For this review, take the finished solid that the model builds, in its own axes (mm). Face numbers are marked on the shaded views. A direction names the side the tool comes from. Give positions to 0.01 mm unless a question says otherwise; leave off trailing zeros. Loops run counter-clockwise (first coordinate to the right, second up) from the corner with the lowest first, then second, coordinate; pieces in that order, holes last. Notation, with made-up numbers: (34.5, 46) - (85.5, 46) arc R33 cw to (85.5, 81) - close; hole circle Ø11 at (64, 81.25). An arc over 180 degrees is marked (long way). Answer as CSV lines item,"result".
from build123d import *

# Parameters (mm, degrees)
EXTRUDE_2_DEPTH = 3
SKETCH_4_R      = 2.5
SKETCH_4_R_2    = 0.95
SKETCH_4_R_3    = 0.973149492
EXTRUDE_5_DEPTH = 6
SKETCH_6_W      = 16
SKETCH_6_H      = 8
EXTRUDE_6_DEPTH = 2.5
EXTRUDE_7_DEPTH = 3.8


with BuildPart() as part:
    # Эскиз1 → Бобышка-Вытянуть2 (new body)
    with BuildSketch(Plane(origin=(0, 0, 0), x_dir=(1, 0, 0), z_dir=(0, 1, 0))):
        with BuildLine():
            Line((-21.078452696, 29.831456886), (2.921547304, 29.831456886))
            ThreePointArc((2.921547304, 29.831456886), (5.042867648, 28.95277723), (5.921547304, 26.831456886))
            Line((5.921547304, 26.831456886), (5.921547304, 2.831456886))
            ThreePointArc((5.921547304, 2.831456886), (5.042867648, 0.710136543), (2.921547304, -0.168543114))
            Line((2.921547304, -0.168543114), (-21.078452696, -0.168543114))
            ThreePointArc((-21.078452696, -0.168543114), (-23.19977304, 0.710136543), (-24.078452696, 2.831456886))
            Line((-24.078452696, 2.831456886), (-24.078452696, 26.831456886))
            ThreePointArc((-24.078452696, 26.831456886), (-23.19977304, 28.95277723), (-21.078452696, 29.831456886))
        make_face()
    extrude(amount=EXTRUDE_2_DEPTH)

    # Эскиз4 → Бобышка-Вытянуть5 (add)
    # profile 1 of 4: a face of its own
    with BuildSketch(Plane.XZ):
        with Locations(Location((1.421547304, -4.831456886, 0), (0, 0, 90))):
            Circle(SKETCH_4_R)
        with Locations(Location((1.421547304, -4.831456886, 0), (0, 0, 270))):
            Circle(SKETCH_4_R_2, mode=Mode.SUBTRACT)
    # profile 2 of 4: a face of its own
    with BuildSketch(Plane.XZ):
        with Locations(Location((-19.578452696, -4.831456886, 0), (0, 0, 90))):
            Circle(SKETCH_4_R)
        with Locations(Location((-19.578452696, -4.831456886, 0), (0, 0, 270))):
            Circle(SKETCH_4_R_3, mode=Mode.SUBTRACT)
    # profile 3 of 4: a face of its own
    with BuildSketch(Plane.XZ):
        with Locations(Location((1.421547304, -17.331456886, 0), (0, 0, 90))):
            Circle(SKETCH_4_R)
        with Locations(Location((1.421547304, -17.331456886, 0), (0, 0, 270))):
            Circle(SKETCH_4_R_2, mode=Mode.SUBTRACT)
    # profile 4 of 4: a face of its own
    with BuildSketch(Plane.XZ):
        with Locations(Location((-19.578452696, -17.331456886, 0), (0, 0, 90))):
            Circle(SKETCH_4_R)
        with Locations(Location((-19.578452696, -17.331456886, 0), (0, 0, 270))):
            Circle(SKETCH_4_R_2, mode=Mode.SUBTRACT)
    extrude(amount=EXTRUDE_5_DEPTH)

    # Эскиз6 → Бобышка-Вытянуть6 (add)
    with BuildSketch(Plane(origin=(0, 3, 0), x_dir=(1, 0, 0), z_dir=(0, 1, 0))):
        with Locations((-9.078452696, 14.831456886)):
            Rectangle(SKETCH_6_W, SKETCH_6_H)
    extrude(amount=EXTRUDE_6_DEPTH)

    # Эскиз7 → Бобышка-Вытянуть7 (add)
    with BuildSketch(Plane(origin=(0, 5.5, 0), x_dir=(1, 0, 0), z_dir=(0, 1, 0))):
        Polygon((-9.078452696, 18.831456886), (-21.578452696, 18.831456886), (-21.578452696, 10.831456886), (3.421547304, 10.831456886), (3.421547304, 18.831456886), align=None)
    extrude(amount=EXTRUDE_7_DEPTH)


solid = part.part
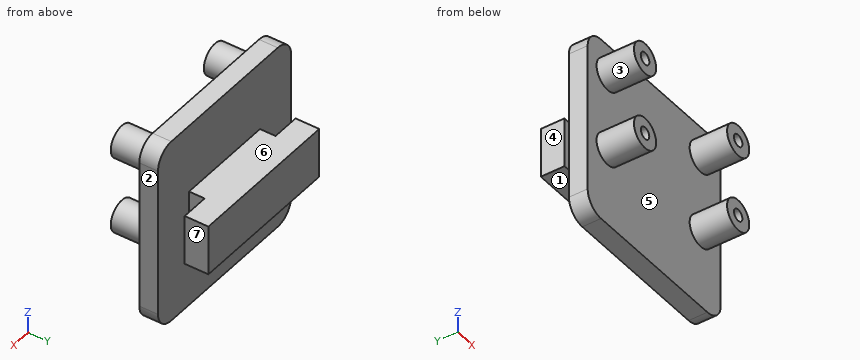
1) Consider section A-A on x = -5. Write out the cut boundary in (y, z), and give its area (3 significant figures).
From the geometry:
outline,"(0, -29.83) - (3, -29.83) - (3, -18.83) - (9.3, -18.83) - (9.3, -10.83) - (3, -10.83) - (3, 0.17) - (0, 0.17) - close"
area,"140 mm^2"
2) Machinability: for the marked faces 1, 2 and 3, which of the approach directions +Z, -Z, +X, -X, +Y, -Y give a long, thin tool a straight path to every point of the face, cutting with its end or side? Answer none if there is none.
From the geometry:
face 1,"-Z, +X, -X, +Y"
face 2,"+Z, -Z, +X, +Y, -Y"
face 3,"-Y"
3) Draft analysis for pull direction X (two halves, no side actions). For the marked faces 4, 5, 6 and 7, state which applies: pulls with the +X half, pulls with the -X half, needs draft (parallel to the pull), parting line crosses it, or undercut.
From the geometry:
face 4,"pulls with the -X half"
face 5,"undercut"
face 6,"needs draft"
face 7,"pulls with the +X half"
4) Consider section D-D on y = 6.25. Write out the cut boundary in (x, z).
From the geometry:
outline,"(-21.58, -18.83) - (3.42, -18.83) - (3.42, -10.83) - (-21.58, -10.83) - close"
5) Consider section B-B on y = -2.25. Write out the cut boundary in (x, z).
From the geometry:
outline,"circle Ø5 at (-19.58, -17.33); circle Ø5 at (-19.58, -4.83); circle Ø5 at (1.42, -17.33); circle Ø5 at (1.42, -4.83); hole circle Ø1.95 at (-19.58, -4.83); hole circle Ø1.9 at (-19.58, -17.33); hole circle Ø1.9 at (1.42, -17.33); hole circle Ø1.9 at (1.42, -4.83)"
6) Insertion check: P1, Ø1.9, axis at y = 6.5, z = -14, coming from the +X side; P2, Ø5, axis at x = 1, z = -13, coming from the -Y side; P3, Ø6, axis at x = -12.5, y = 7.5, coming from the -Z side; P4, Ø1.5, axis at x = -1, z = -9.5, coming from the -Y side. Each pin has a flat end and moves straight along its axis. Give the tip position at first contact, or say it passes through.
From the geometry:
P1,"stops at x = 3.42"
P2,"stops at y = -6"
P3,"stops at z = -18.83"
P4,"stops at y = 0"
7) Consider section C-C on z = -11.5. Write out the cut boundary in (x, y).
From the geometry:
outline,"(-24.08, 0) - (5.92, 0) - (5.92, 3) - (-1.08, 3) - (-1.08, 5.5) - (3.42, 5.5) - (3.42, 9.3) - (-21.58, 9.3) - (-21.58, 5.5) - (-17.08, 5.5) - (-17.08, 3) - (-24.08, 3) - close"
8) Wall thickness on line 1 (X direction, y = -2.25, z = -18); line 2 (Y direction, x = -9, z = -15.5); line 3 (Y direction, x = -13.5, z = -5.5): over which ranges is each line inside the solid? List them lowest first. Write a range as from..to.
From the geometry:
line 1,"x = -21.99..-20.25, -18.9..-17.17, -0.99..0.75, 2.1..3.83"
line 2,"y = 0..9.3"
line 3,"y = 0..3"
